from build123d import *

# Parameters (mm, degrees)
SKETCH1_W           = 35
SKETCH1_H           = 0.7
SKETCH1_H_2         = 35
BOSS_EXTRUDE1_DEPTH = 5
CHAMFER1_SIZE       = 3
SKETCH4_R           = 2.6
SKETCH4_R_2         = 1.58
BOSS_EXTRUDE2_DEPTH = 1


with BuildPart() as part:
    # Sketch1 → Boss-Extrude1 (new body)
    with BuildSketch(Plane(origin=(0, 0, 0), x_dir=(1, 0, 0), z_dir=(0, 1, 0))):
        with BuildLine():
            Line((7.5, 17.5), (13.1, 17.5))
            Line((13.1, 17.5), (13.1, 30))
            Line((13.1, 30), (7.5, 30))
            Line((7.5, 30), (7.5, 25.524823935))
            ThreePointArc((7.5, 25.524823935), (8.018677324, 24.703939201), (8.2, 23.75))
            ThreePointArc((8.2, 23.75), (8.018677324, 22.796060799), (7.5, 21.975176065))
            Line((7.5, 21.975176065), (7.5, 17.5))
        make_face()
        with BuildLine():
            Line((-1.9, 30), (-1.9, 17.5))
            Line((-1.9, 17.5), (7.5, 17.5))
            Line((7.5, 17.5), (7.5, 21.975176065))
            ThreePointArc((7.5, 21.975176065), (3, 23.75), (7.5, 25.524823935))
            Line((7.5, 25.524823935), (7.5, 30))
            Line((7.5, 30), (-1.9, 30))
        make_face()
        with Locations((0, -17.85)):
            Rectangle(SKETCH1_W, SKETCH1_H)
        Rectangle(SKETCH1_W, SKETCH1_H_2)
    extrude(amount=BOSS_EXTRUDE1_DEPTH)

    # Chamfer1
    chamfer1_edges = [part.edges().sort_by_distance(p)[0] for p in [
        (-1.9, 2.5, -30),
        (13.1, 2.5, -30),
        (17.5, 2.5, -17.5),
        (17.5, 2.5, 18.2),
        (-17.5, 2.5, 18.2),
        (-17.5, 2.5, -17.5),
    ]]
    chamfer(chamfer1_edges, length=CHAMFER1_SIZE)

    # Sketch4 → Boss-Extrude2 (add)
    with BuildSketch(Plane(origin=(0, 0.3, 0), x_dir=(1, 0, 0), z_dir=(0, 1, 0))):
        with Locations((5.6, 23.75)):
            Circle(SKETCH4_R)
        with Locations((5.6, 23.75)):
            Circle(SKETCH4_R_2, mode=Mode.SUBTRACT)
    extrude(amount=BOSS_EXTRUDE2_DEPTH)


solid = part.part
Read the model definition and answer for the solid it produces. Units are mm, in the model's axes. A direction names the side the tool comes from. Round coordinates to 2 decimals unless told otherwise and drop trailing zeros. Order: outer loops, then holes, each group sorted by start corner. A loop starts at its lowest first (then second) coordinate and runs counter-clockwise, first axis right, second up. Notation, with made-up numbers: (1.25, 43) - (36.25, 43) arc R6 ccw to (36.25, 54) - close; hole circle Ø3 at (-12, 1.25). An arc over 180 degrees is marked (long way). Use one line per item in the form item = value. Start each with the question number.
(1) Flat-ended cylindrical pins translate along their axes: pin 1 Ø3 at (x, z) = (5.6, -23.75) entering from -Y; pin 2 Ø1.5 at (x, y) = (13.5, 3) entering from -Z; pin 3 Ø7 at (x, z) = (5.6, -23.75) entering from -Y; pin 4 Ø1.6 at (x, z) = (4.5, -25) entering from -Y. Find the tip coordinate at first contact, or state that the pin passes through.
(2) The part is cut by section C-C (z = -16). Give the vertices of the cut face in (x, y).
(3) For faces 1 (the face through (14, 2, -17.5)), 2 (the face through (-1.9, 2, -22)), 3 (the face through (6, 0.3, -22)), determine the directions among +Z, -Z, +X, -X, +Y, -Y from which every point of the face is accessible in a straight line to the end or side of a thin tool.
(4) The part is cut by section A-A (x = 5.6). Give the vertices of the cut face in (y, z), then the cut area to 3 significant figures.
(5) The part is cut by section B-B (y = 2.5). Give the vertices of the cut face in (x, z), then the cut area to 3 significant figures.
(6) The part is cut by section D-D (x = 11). Give the vertices of the cut face in (y, z), then the cut area to 4 significant figures.
(7) Determine the mould class of faces 4 (the face through (0, 5, -1)), 5 (the face through (-8, 2, -17.5)), 6 (the face through (5.3, 0.8, -22.2)) for opening direction Z: +Z half, -Z half, draft (parallel to the pull), parting line (faces both ways), or undercut.
(8) Find the intervals of material crossed by line 1 along Z through (x, y) = (5.6, 2.9); line 2 along X through (y, z) = (1, -23.75); line 3 along Z through (x, y) = (-7.5, 3.5), in increasing order. Write a range as from..to.
Checked values:
q1.pin_1 = through
q1.pin_2 = -27.35
q1.pin_3 = 0
q1.pin_4 = 0.3
q2.outline = (-16, 0) - (16, 0) - (16, 5) - (-16, 5) - close
q3.face_1 = -Z, +X, +Y, -Y
q3.face_2 = -Z, -X, +Y, -Y
q3.face_3 = -Y
q4.outline = (0, -30) - (5, -30) - (5, -26.35) - (1.3, -26.35) - (1.3, -25.33) - (0.3, -25.33) - (0.3, -26.35) - (0, -26.35) - close; (0, -21.15) - (0.3, -21.15) - (0.3, -22.17) - (1.3, -22.17) - (1.3, -21.15) - (5, -21.15) - (5, 18.2) - (0, 18.2) - close
q4.area = 217 mm^2
q5.outline = (-17.5, -14.5) - (-14.5, -17.5) - (-1.9, -17.5) - (-1.9, -27) - (1.1, -30) - (10.1, -30) - (13.1, -27) - (13.1, -17.5) - (14.5, -17.5) - (17.5, -14.5) - (17.5, 15.2) - (14.5, 18.2) - (-14.5, 18.2) - (-17.5, 15.2) - close; hole circle Ø5.2 at (5.6, -23.75)
q5.area = 1,390 mm^2
q6.outline = (0, -29.1) - (5, -29.1) - (5, 18.2) - (0, 18.2) - close
q6.area = 236.5 mm^2
q7.face_4 = draft
q7.face_5 = -Z half
q7.face_6 = undercut
q8.line_1 = -30..-26.35, -21.15..18.2
q8.line_2 = -1.9..4.02, 7.18..13.1
q8.line_3 = -17.5..18.2
